Verification items for the finished model (mm, model axes). A direction names the side the tool comes from. Give positions to 0.01 mm unless a question says otherwise; leave off trailing zeros. Write each loop counter-clockwise with the first axis right and the second up, starting at its lowest first coordinate (ties: lowest second). Pieces come first, ordered by that corner, then holes. Notation, with made-up numbers: M -2.5,17 L 14.5,17 A20 cw 14.5,55 Z; hole C 85.25,18 d1. An arc over 180 degrees is marked long. Answer as a JSON object with one key per item and string values.
Autodesk Inventor part; units mm, degrees
ref_plane "YZ Plane" through (0, 0, 0) normal (1, 0, 0) x (0, 1, 0)
ref_plane "XZ Plane" through (0, 0, 0) normal (0, 1, 0) x (-1, 0, 0)
ref_plane "XY Plane" through (0, 0, 0) normal (0, 0, 1) x (1, 0, 0)
sketch "Sketch1" plane through (0, 0, 0) normal (0, 0, 1) x (1, 0, 0)
  line L0 (-60, 40) -> (60, 40)
  line L1 (60, 40) -> (60, -40)
  line L2 (60, -40) -> (-60, -40)
  line L3 (-60, -40) -> (-60, 40)
  point P0 (0, 0)
  point P1 (0, 40)
  point P2 (-60, 0)
  dimension "d0" = 120
  dimension "d1" = 80
extrude "Extrusion1" add sketch "Sketch1" along normal blind 80
sketch "Sketch2" plane through (-60, -40, 0) normal (-1, 0, 0) x (0, 0, 1)
  line L0 (60, 60) -> (20, 60)
  line L1 (20, 60) -> (20, 20)
  line L2 (20, 20) -> (60, 20)
  line L3 (60, 20) -> (60, 60)
  line L4 (0, 0) -> (0, 80)
  line L5 (0, 80) -> (80, 80)
  point P0 (0, 40)
  point P1 (60, 40)
  point P2 (0, 40)
  point P3 (40, 60)
  point P4 (40, 80)
  dimension "d4" = 40
  dimension "d5" = 40
extrude "Extrusion2" add sketch "Sketch2" along normal blind 30
sketch "Sketch3" plane through (60, -40, 0) normal (1, 0, 0) x (0, 0, -1)
  line L0 (-50, 25) -> (-30, 25)
  line L1 (-30, 25) -> (-30, 55)
  line L2 (-30, 55) -> (-50, 55)
  line L3 (-50, 55) -> (-50, 25)
  line L4 (0, 0) -> (-80, 0)
  line L5 (-80, 0) -> (-80, 80)
  line L6 (-38, 33) -> (-42, 33)
  line L7 (-42, 33) -> (-42, 28)
  line L8 (-42, 28) -> (-38, 28)
  line L9 (-38, 28) -> (-38, 33)
  line L10 (-37, 40) -> (-43, 40)
  line L11 (-43, 40) -> (-43, 36)
  line L12 (-43, 36) -> (-37, 36)
  line L13 (-37, 36) -> (-37, 40)
  line L14 (-37, 46) -> (-43, 46)
  line L15 (-43, 46) -> (-43, 42)
  line L16 (-43, 42) -> (-37, 42)
  line L17 (-37, 42) -> (-37, 46)
  line L18 (-44, 49) -> (-36, 49)
  line L19 (-36, 49) -> (-36, 52)
  line L20 (-36, 52) -> (-44, 52)
  line L21 (-44, 52) -> (-44, 49)
  point P0 (0, 40)
  point P1 (-40, 25)
  point P2 (-40, 0)
  point P3 (-50, 40)
  point P4 (-80, 40)
  point P5 (-40, 28)
  point P6 (-40, 36)
  point P7 (-40, 42)
  point P8 (-40, 52)
  point P9 (-40, 55)
  dimension "d21" = 30
  dimension "d20" = 20
  dimension "d19" = 5
  dimension "d18" = 4
  dimension "d16" = 4
  dimension "d15" = 6
  dimension "d13" = 6
  dimension "d12" = 4
  dimension "d9" = 3
  dimension "d10" = 8
  dimension "d14" = 3
  dimension "d11" = 2
  dimension "d8" = 3
  dimension "d17" = 3
extrude "Extrusion3" cut sketch "Sketch3" against normal blind 5
sketch "Sketch4" plane through (0, 0, 80) normal (0, 0, 1) x (1, 0, 0)
  circle A0 centre (55, 35) radius 2.5
  line L0 (60, 40) -> (-60, 40)
  line L1 (60, -40) -> (60, 40)
  circle A1 centre (55, -35) radius 2.5
  circle A2 centre (-55, 35) radius 2.5
  circle A3 centre (-55, -35) radius 2.5
  point P0 (0, 0)
  dimension "d25" = 5
  dimension "d26" = 5
  dimension "d27" = 5
  dimension "d30" = 70
  dimension "d33" = 110
extrude "Extrusion4" cut sketch "Sketch4" against normal blind 5
properties part number "prismatic"
1) Section check C-C on z = 11.5. Record the boundary of the cut face in (x, y).
Completed:
{"outline": "M -60,-40 L 60,-40 L 60,40 L -60,40 Z"}
2) Section check A-A on y = 35. Record the boundary of the cut face in (x, z).
Completed:
{"outline": "M -60,0 L 60,0 L 60,80 L 57.5,80 L 57.5,75 L 52.5,75 L 52.5,80 L -52.5,80 L -52.5,75 L -57.5,75 L -57.5,80 L -60,80 Z"}
3) Access from +Z, -Z, +X, -X, +Y, -Y to the whole of each face (thin tool, end or side, straight path). Record for faces 4 (the face through (-75, -20, 40)), 5 (the face through (55, 35, 75)), 6 (the face through (-75, 0, 60)).
Completed:
{"face 4": "+Z, -Z, -X, -Y", "face 5": "+Z", "face 6": "+Z, -X, +Y, -Y"}
4) Go/stop test with a flat-tipped pin: pin 1 (1 mm diameter, centred on x = -69, z = 39, fed in from +Y). Record where the tip stops, or that it passes through.
Completed:
{"pin 1": "stops at y = 20"}
5) Thickness scan on L1, parallel to Y at x = 55, z = 76.8; L2, parallel to X at y = -15.5, z = 4.5; L3, parallel to Y at x = -77.5, z = 30. Record the ranges inside material, lowest first.
Completed:
{"L1": "y = -40 to -37.5, -32.5 to 32.5, 37.5 to 40", "L2": "x = -60 to 60", "L3": "y = -20 to 20"}
6) Release check for a two-part mould opening along X. For faces 1 (the face through (-55, 35, 75)), 2 (the face through (60, 11, 40)), 3 (the face through (-1, 1, 0)) record: pulls with the +X half, pulls with the -X half, needs draft (parallel to the pull), parting line crosses it, or undercut.
Completed:
{"face 1": "undercut", "face 2": "pulls with the +X half", "face 3": "needs draft"}
7) Section check B-B on x = -75.5. Record the boundary of the cut face in (y, z).
Completed:
{"outline": "M -20,20 L 20,20 L 20,60 L -20,60 Z"}
